Geometry: final body of the model. Coordinates: model frame, mm. Face numbers are marked on the shaded views. Give positions to 0.01 mm unless a question says otherwise; leave off trailing zeros. Write each loop counter-clockwise with the first axis right and the second up, starting at its lowest first coordinate (ties: lowest second). Pieces come first, ordered by that corner, then holes. Notation, with made-up numbers: (57.25, -36) -> (94.25, -36) arc R10 cw to (94.25, -28) -> close; hole circle Ø2 at (44, 42.5). An arc over 180 degrees is marked (long way). Answer as a JSON object with one key per item and string values. Group by question number.
(1) Material intervals for probe 1 along Y at (x, z) = (0, 118); probe 2 along Y at (x, z) = (-28, 36.5); probe 3 along X at (y, z) = (-31, 153), sorted ascending.
(2) Draft query along Y for the marked faces 1, 2 and 3. Return one class per face: +Y half, -Y half, draft (parallel to the pull), parting line (faces both ways), or undercut.
(3) Section query A-A on x = 0. Output: boundary loops of the cut face in (y, z), plus the area to 3 significant figures.
(4) Section query C-C on z = 148.5. Output: boundary loops of the cut face in (x, y).
(5) Contact query for flat-ended pins moving along their axis: pin 1 Ø1 at (x, z) = (-23.5, 42.5) entering from -Y; pin 2 Ø4 at (x, z) = (9.5, 123.5) entering from +Y; pin 3 Ø6 at (x, z) = (47.5, 48.5) entering from -Y. Output: stop coordinate, or through.
(6) Section query D-D on y = 59. Output: boundary loops of the cut face in (x, z).
from build123d import *

# Parameters (mm, degrees)
F0_R     = 74.2865291694
F1_DEPTH = 151.892
F2_DEPTH = 53.594
F3_R     = 54.1549709352
F4_DEPTH = 195.58
F5_DEPTH = 92.202


# Not quite as in the source:
# - a feature names something its author has since deleted; it is built from what else it names


with BuildPart() as f1:
    # F0 (on Top) → F1 (new body)
    with BuildSketch(Plane.XY):
        Circle(F0_R)
    extrude(amount=F1_DEPTH)

    # F2 (add): a face of the model
    f2_faces = [f1.faces().sort_by_distance(p)[0] for p in [
        (0, 0, 151.892),
    ]]
    extrude(f2_faces, amount=F2_DEPTH)

    # F3 (on face) → F4 (cut)
    with BuildSketch(Plane.XY.offset(205.486)):
        Circle(F3_R)
    extrude(amount=-F4_DEPTH, mode=Mode.SUBTRACT)

    # F5 (cut): a face of the model
    f5_faces = [f1.faces().sort_by_distance(p)[0] for p in [
        (0, 0, 9.906),
    ]]
    extrude(f5_faces, amount=-F5_DEPTH, mode=Mode.SUBTRACT)


solid = f1.part
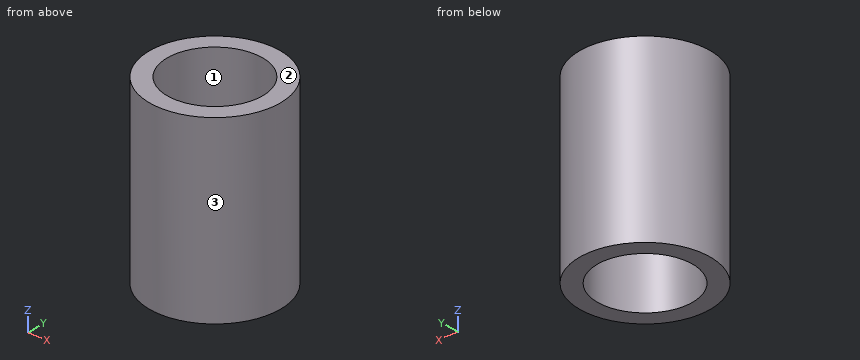
Answer list:
{
 "1": {"probe 1": "-74.29 to -54.15, 54.15 to 74.29", "probe 2": "-68.81 to -46.35, 46.35 to 68.81", "probe 3": "-67.51 to -44.4, 44.4 to 67.51"},
 "2": {"face 1": "undercut", "face 2": "draft", "face 3": "parting line"},
 "3": {"outline": "(-74.29, 0) -> (-54.15, 0) -> (-54.15, 205.49) -> (-74.29, 205.49) -> close; (54.15, 0) -> (74.29, 0) -> (74.29, 205.49) -> (54.15, 205.49) -> close", "area": "8,270 mm2"},
 "4": {"outline": "circle Ø148.57 at (0, 0); hole circle Ø108.31 at (0, 0)"},
 "5": {"pin 1": "y = -70.64", "pin 2": "y = 73.91", "pin 3": "y = -59.48"},
 "6": {"outline": "(-45.14, 0) -> (45.14, 0) -> (45.14, 205.49) -> (-45.14, 205.49) -> close"}
}
